The listing builds one solid part. Answer for the finished solid, in the listing's coordinates (mm). A direction names the side the tool comes from. Give positions to 0.01 mm unless a question says otherwise; leave off trailing zeros. Loops run counter-clockwise (first coordinate to the right, second up) from the corner with the lowest first, then second, coordinate; pieces in that order, holes last. Notation, with made-up numbers: M 16,49 L 27,49 A28 ccw 27,85 Z; hole C 86,11.5 d2. An arc over 180 degrees is marked long. Return JSON: item names as keys, results as strings.
from build123d import *

# Parameters (mm, degrees)
F0_R     = 16.5
F1_DEPTH = 31.5
F2_DEPTH = 17.5
F4_DEPTH = 19.7
F3_R     = 5
F5_DEPTH = 3
F6_D     = 3.3
F6_DEPTH = 6
F6_TIP   = 0.9914200214


with BuildPart() as f1:
    # F0 (on Front) → F1 (new body)
    with BuildSketch(Plane.XZ):
        Circle(F0_R)
    extrude(amount=F1_DEPTH)

    # F2 (add): a face of the model
    f2_faces = [f1.faces().sort_by_distance(p)[0] for p in [
        (0, 0, 0),
    ]]
    extrude(f2_faces, amount=F2_DEPTH)

    # F3 (on face) → F4 (join)
    with BuildSketch(Plane.XZ.offset(31.5)):
        with BuildLine():
            ThreePointArc((-2.5, -1.6583123952), (0.8660254038, -2.8722813233), (3, 0))
            ThreePointArc((3, 0), (0.8660254038, 2.8722813233), (-2.5, 1.6583123952))
            Line((-2.5, 1.6583123952), (-2.5, -1.6583123952))
        make_face()
    extrude(amount=F4_DEPTH)

    # F3 (on face) → F5 (join)
    with BuildSketch(Plane.XZ.offset(31.5)):
        Circle(F3_R)
        with BuildLine():
            ThreePointArc((-2.5, 1.6583123952), (0.8660254038, 2.8722813233), (3, 0))
            ThreePointArc((3, 0), (0.8660254038, -2.8722813233), (-2.5, -1.6583123952))
            ThreePointArc((-2.5, -1.6583123952), (-3, 0), (-2.5, 1.6583123952))
        make_face(mode=Mode.SUBTRACT)
        with BuildLine():
            Line((-2.5, -1.6583123952), (-2.5, 1.6583123952))
            ThreePointArc((-2.5, 1.6583123952), (-3, 0), (-2.5, -1.6583123952))
        make_face()
    extrude(amount=F5_DEPTH)

    # F6
    with Locations(Plane.XZ.offset(31.5)):
        with Locations((11, 0), (0, -11), (0, 11), (-11, 0)):
            Hole(F6_D / 2, depth=F6_DEPTH)
            with Locations((0, 0, -(F6_DEPTH + F6_TIP / 2))):  # 118° drill point
                Cone(0, F6_D / 2, F6_TIP, mode=Mode.SUBTRACT)


solid = f1.part
(1) The part is cut by section A-A (y = -47). Determine the outline of the cut face in (x, z).
Values follow:
{"outline": "M -2.5,-1.66 A3 ccw long -2.5,1.66 Z"}
(2) Given pin 1 (4 mm diameter, centred on x = 7.5, y = -20.5, fed in from +Z); pin 2 (4 mm diameter, centred on y = 0.5, z = -11, fed in from +X); pin 3 (8 mm diameter, centred on x = 2.5, y = -41.5, fed in from -Z), each flat-ended and moving along its own axis, determine where each tip first touches the part or whether it passes through.
Values follow:
{"pin 1": "z = 15.56", "pin 2": "x = 13.83", "pin 3": "z = -3"}
(3) Determine the mould class of faces 3 (the flat face through (-2.5, -43, 0)), 4 (the flat face through (0, 17.5, 0)), 5 (the cylindrical face through (-1.08, -32.98, -4.88)), 6 (the conical face through (-0.04, -24.68, 11.28)) for opening direction X: released by +X, released by -X, zero draft, split by the parting line, or undercut.
Values follow:
{"face 3": "released by -X", "face 4": "zero draft", "face 5": "split by the parting line", "face 6": "undercut"}
(4) A tool of negligible diameter and unlimited length cuts with its end or side. For faces 1 (the cylindrical face through (15.24, -7.34, -6.32)), 2 (the flat face through (-0.1, -34.5, -3.3)), from which of +Z, -Z, +X, -X, +Y, -Y can it reach the whole face along a straight path? Write none if from no direction.
Values follow:
{"face 1": "+Y, -Y", "face 2": "-Y"}
(5) Straight lines are drawn through the part: line 1 along Z through (x, y) = (0, -28.3); line 2 along X through (y, z) = (10, 0.5); line 3 along Y through (x, z) = (9.5, 6.5). For each, find the intervals that lie inside material, in ascending order.
Values follow:
{"line 1": "-16.5 to -12.65, -9.35 to 9.35, 12.65 to 16.5", "line 2": "-16.49 to 16.49", "line 3": "-31.5 to 17.5"}
(6) The part is cut by section B-B (x = -8.5). Determine the outline of the cut face in (y, z), and give its area (3 significant figures).
Values follow:
{"outline": "M -31.5,-14.14 L 17.5,-14.14 L 17.5,14.14 L -31.5,14.14 Z", "area": "1,390 mm²"}
